Job drawing, mm, ordinate dimensions from the low corner. One solid piece. Coordinates: 2 decimals unless noted, no trailing zeros. Loops run counter-clockwise (first coordinate to the right, second up) from the corner with the lowest first, then second, coordinate; pieces in that order, holes last. Notation, with made-up numbers: M 14.5,8.5 L 34.5,8.5 A14 ccw 34.5,30.5 Z; hole C 50.25,-39 d3. An arc over 180 degrees is marked long. Write each question's results on one line, items separated by ' | '. Start each with the question number.
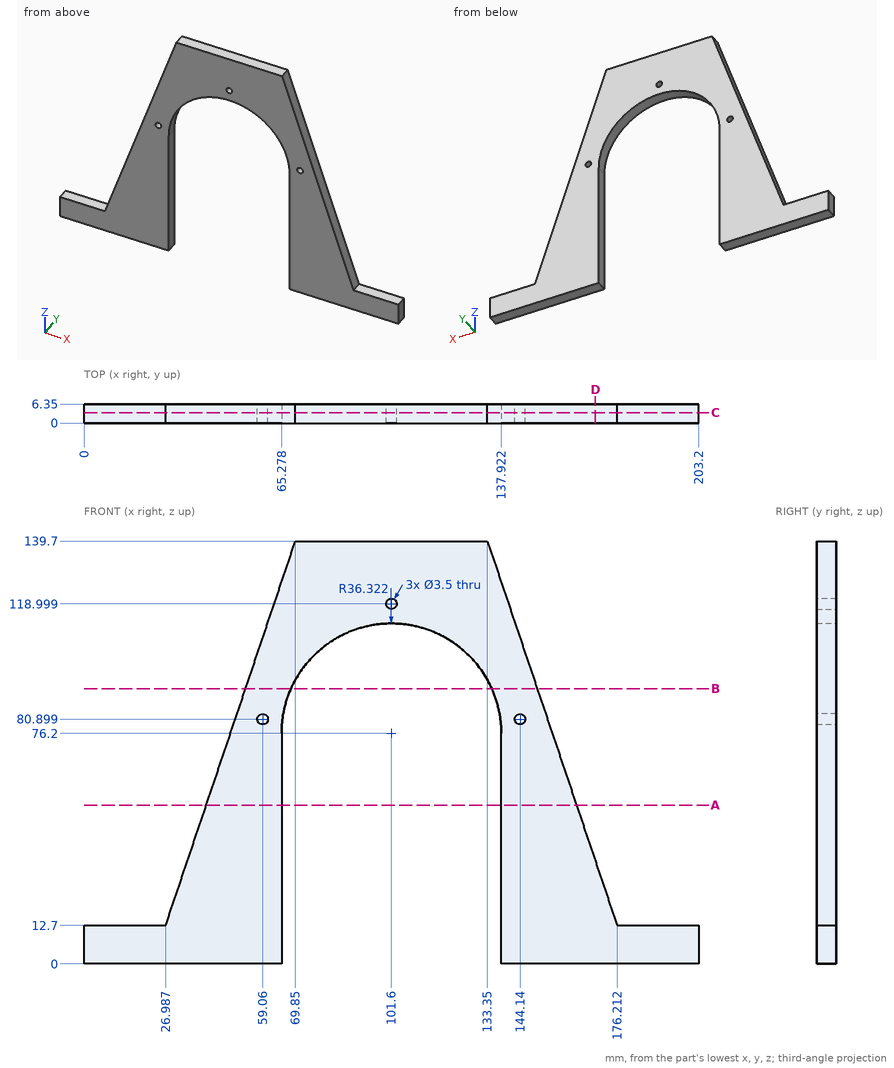
1. Band-saw the part on A-A, the plane z = 52.5. List the corners of the cut face in (x, y).
2. Band-saw the part on B-B, the plane z = 91. List the corners of the cut face in (x, y).
3. Pin check, flat tips, straight feed: pin 1 (4 mm diameter, centred on x = 101.6, z = 118.999, fed in from -Y); pin 2 (3 mm diameter, centred on x = 187.5, y = 3, fed in from +Z); pin 3 (1.5 mm diameter, centred on y = 1.5, z = 89.5, fed in from +X) (1 decimal); pin 4 (3 mm diameter, centred on y = 1, z = 116.5, fed in from -X). Stop position of each tip, or through.
4. Wall check: line 1 along X through (y, z) = (3.25, 6); line 2 along X through (y, z) = (3.5, 81) (1 decimal); line 3 along Z through (x, y) = (17, 5.25). Give the ranges that are in metal, low to high.
5. Band-saw the part on C-C, the plane y = 3.5. Give the number of separate pieces and of enclosed holes in the cut face, plus the area to 3 significant figures.
6. Band-saw the part on D-D, the plane x = 169. List the corners of the cut face in (y, z), plus the area to 3 significant figures.
Checked values:
1) outline: M 40.42,0 L 65.28,0 L 65.28,6.35 L 40.42,6.35 Z; M 137.92,0 L 162.78,0 L 162.78,6.35 L 137.92,6.35 Z
2) outline: M 53.41,0 L 68.43,0 L 68.43,6.35 L 53.41,6.35 Z; M 134.77,0 L 149.79,0 L 149.79,6.35 L 134.77,6.35 Z
3) pin 1: y = 0 | pin 2: z = 12.7 | pin 3: x = 150.5 | pin 4: x = 61.51
4) line 1: 0 to 65.28, 137.92 to 203.2 | line 2: 50 to 57.3, 60.8 to 65.6, 137.6 to 142.4, 145.9 to 153.2 | line 3: 0 to 12.7
5) separate pieces: 1 | enclosed holes: 3 | area: 8,450 mm²
6) outline: M 0,0 L 6.35,0 L 6.35,34.07 L 0,34.07 Z | area: 216 mm²
